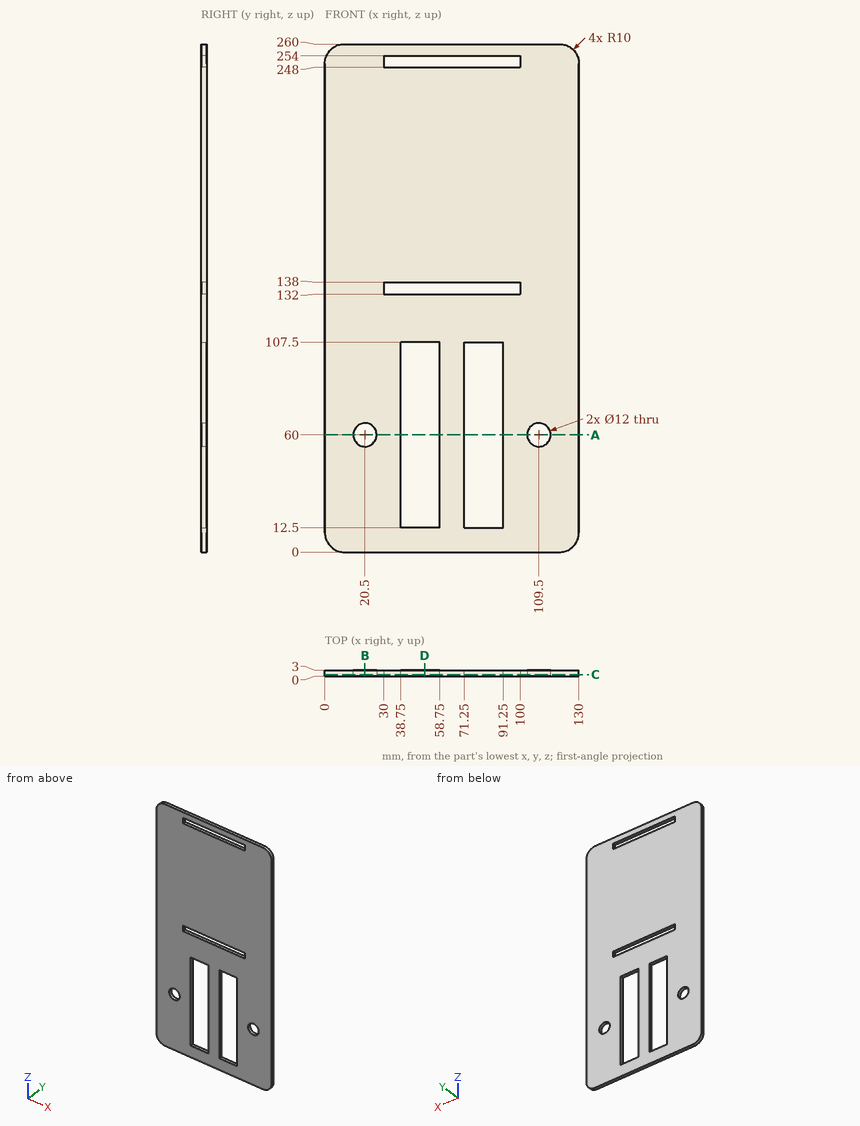
Can you work these out from the drawing? Everything is in mm from the part's minimum corner. Give positions to 0.01 mm unless a question says otherwise; leave off trailing zeros. Loops run counter-clockwise (first coordinate to the right, second up) from the corner with the lowest first, then second, coordinate; pieces in that order, holes last. Notation, with made-up numbers: (-21, 5) -> (36, 5) arc R14 ccw to (36, 24) -> close; hole circle Ø4 at (47, 82). An arc over 180 degrees is marked (long way). Write item = value, one per line.
1) Suppose I cut it at C-C on y = 0.65. Write out the boundary of the cut face in (x, z).
Check result:
outline = (0, 10) arc R10 ccw to (10, 0) -> (120, 0) arc R10 ccw to (130, 10) -> (130, 250) arc R10 ccw to (120, 260) -> (10, 260) arc R10 ccw to (0, 250) -> close; hole circle Ø12 at (20.5, 60); hole (30, 132) -> (100, 132) -> (100, 138) -> (30, 138) -> close; hole (30, 248) -> (100, 248) -> (100, 254) -> (30, 254) -> close; hole (38.75, 12.5) -> (58.75, 12.5) -> (58.75, 107.5) -> (38.75, 107.5) -> close; hole (71.25, 12.5) -> (91.25, 12.5) -> (91.25, 107.5) -> (71.25, 107.5) -> close; hole circle Ø12 at (109.5, 60)
2) I need wall thicknesses on L1, parallel to X at y = 1.3, z = 99; L2, parallel to Z at x = 31.5, y = 2.7; L3, parallel to Z at x = 20.5, y = 0.6. Which ranges of each line are inside material? Lowest first, please. Write a range as from..to.
Check result:
L1 = 0..38.75, 58.75..71.25, 91.25..130
L2 = 0..132, 138..248, 254..260
L3 = 0..54, 66..260
3) Suppose I cut it at D-D on x = 51. Write out the boundary of the cut face in (y, z).
Check result:
outline = (0, 0) -> (3, 0) -> (3, 12.5) -> (0, 12.5) -> close; (0, 107.5) -> (3, 107.5) -> (3, 132) -> (0, 132) -> close; (0, 138) -> (3, 138) -> (3, 248) -> (0, 248) -> close; (0, 254) -> (3, 254) -> (3, 260) -> (0, 260) -> close
4) Suppose I cut it at A-A on z = 60. Write out the boundary of the cut face in (x, y).
Check result:
outline = (0, 0) -> (14.5, 0) -> (14.5, 3) -> (0, 3) -> close; (26.5, 0) -> (38.75, 0) -> (38.75, 3) -> (26.5, 3) -> close; (58.75, 0) -> (71.25, 0) -> (71.25, 3) -> (58.75, 3) -> close; (91.25, 0) -> (103.5, 0) -> (103.5, 3) -> (91.25, 3) -> close; (115.5, 0) -> (130, 0) -> (130, 3) -> (115.5, 3) -> close
5) Suppose I cut it at B-B on x = 20.5. Write out the boundary of the cut face in (y, z), then the cut area to 3 significant figures.
Check result:
outline = (0, 0) -> (3, 0) -> (3, 54) -> (0, 54) -> close; (0, 66) -> (3, 66) -> (3, 260) -> (0, 260) -> close
area = 744 mm2
